Here's how the part is built. I have some questions about the finished solid (model axes, mm). Face numbers are marked on the shaded views. A direction names the side the tool comes from. Give positions to 0.01 mm unless a question says otherwise; leave off trailing zeros. Loops run counter-clockwise (first coordinate to the right, second up) from the corner with the lowest first, then second, coordinate; pieces in that order, holes last. Notation, with made-up numbers: (-5.5, 14.25) - (29.5, 14.25) arc R25 cw to (29.5, 29.25) - close; hole circle Ø3 at (-3, 62.5). An arc over 180 degrees is marked (long way). Put each result on its own line as item: value. Start each with the question number.
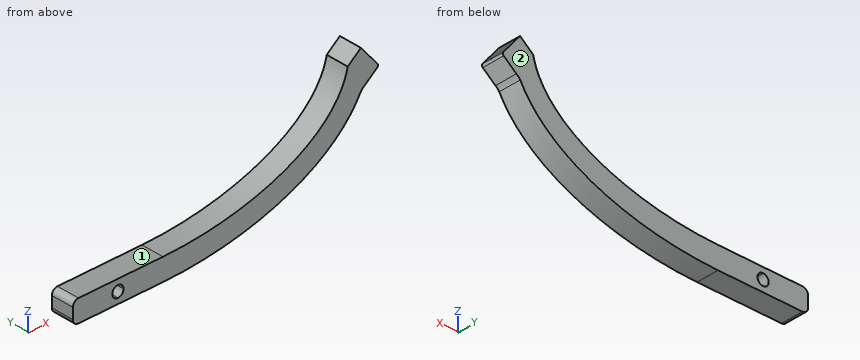
from build123d import *

# Parameters (mm, degrees)
F1_DEPTH = 10


# Not quite as in the source:
# - ends of sketch curves that miss each other by under 0.0002 mm in the source are joined
# - the dataset's text gives a spline's control points without its knots; the knots are read off the source's solid


with BuildPart() as f1:
    # F0 (on Front) → F1 (new body)
    with BuildSketch(Plane.XZ):
        with BuildLine():
            Line((-65.2858525045, 19.1747198819), (-82.7858525045, 19.1747198819))
            ThreePointArc((-82.7858525045, 19.1747198819), (-84.5536194575, 18.4424868349), (-85.2858525045, 16.6747198819))
            Line((-85.2858525045, 16.6747198819), (-85.2858525045, 11.9747207331))
            ThreePointArc((-85.2858525045, 11.9747207331), (-84.5536194575, 10.2069537801), (-82.7858525045, 9.4747207331))
            Line((-82.7858525045, 9.4747207331), (-65.2858525045, 9.4747207331))
            Line((-65.2858525045, 9.4747207331), (-65.2858525045, 11.8247203075))
            ThreePointArc((-65.2858525045, 11.8247203075), (-67.7858525045, 14.3247203075), (-65.2858525045, 16.8247203075))
            Line((-65.2858525045, 16.8247203075), (-65.2858525045, 19.1747198819))
        make_face()
        with BuildLine():
            Line((-45.2858542078, 19.1747198819), (-65.2858525045, 19.1747198819))
            Line((-65.2858525045, 19.1747198819), (-65.2858525045, 16.8247203075))
            ThreePointArc((-65.2858525045, 16.8247203075), (-63.5180855515, 16.0924872605), (-62.7858525045, 14.3247203075))
            ThreePointArc((-62.7858525045, 14.3247203075), (-63.5180855515, 12.5569533545), (-65.2858525045, 11.8247203075))
            Line((-65.2858525045, 11.8247203075), (-65.2858525045, 9.4747207331))
            Line((-65.2858525045, 9.4747207331), (-45.2858525045, 9.4747207331))
            Line((-45.2858525045, 9.4747207331), (-45.2858542078, 19.1747198819))
        make_face()
        with BuildLine():
            add(Edge.make_bspline(
                [(-45.2858542078, 19.1747198819), (-7.4020708747, 19.1747265342), (31.6102094948, 32.6948724687), (36.8064381182, 57.2929121554)],
                knots=[0, 0, 0, 0, 90.5104471403, 90.5104471403, 90.5104471403, 90.5104471403], degree=3))
            Line((-45.2858542078, 19.1747198819), (-45.2858525045, 9.4747207331))
            add(Edge.make_bspline(
                [(-45.2858525045, 9.4747207331), (-40.2618978901, 9.4747216153), (-30.1894784684, 9.9223917761), (-15.362918013, 11.9100905112), (-1.1709415961, 15.2094571968), (12.0418148644, 19.8491680066), (21.9570020274, 24.9039048155), (29.047465051, 29.7583646646), (33.8850587667, 33.8431124408), (38.1663250739, 38.413322434), (40.9420261226, 42.3174471625), (42.2861221075, 44.6734195955), (42.5837097689, 45.2249895308)],
                knots=[0, 0, 0, 0, 0.125, 0.25, 0.375, 0.5, 0.625, 0.6875, 0.75, 0.8125, 0.875, 0.8937572345, 0.8937572345, 0.8937572345, 0.8937572345], degree=3))
            add(Edge.make_bspline(
                [(42.5837097689, 45.2249895308), (42.9712246909, 45.9432369861), (43.3372375793, 46.6745796576), (43.6802036603, 47.4185139687)],
                knots=[0.8937572345, 0.8937572345, 0.8937572345, 0.8937572345, 0.9181826701, 0.9181826701, 0.9181826701, 0.9181826701], degree=3))
            Line((43.6802036603, 47.4185139687), (44.295853648, 46.8606554446))
            Line((44.295853648, 46.8606554446), (49.9209338751, 51.373229087))
            ThreePointArc((49.9209338751, 51.373229087), (50.2893303324, 52.0452304101), (50.0738615656, 52.7806724123))
            Line((50.0738615656, 52.7806724123), (42.6465372943, 61.9985727481))
            Line((42.6465372943, 61.9985727481), (36.8064381182, 57.2929121554))
        make_face()
        with BuildLine():
            add(Edge.make_bspline(
                [(42.5837097689, 45.2249895308), (42.9712246909, 45.9432369861), (43.3372375793, 46.6745796576), (43.6802036603, 47.4185139687)],
                knots=[0.8937572345, 0.8937572345, 0.8937572345, 0.8937572345, 0.9181826701, 0.9181826701, 0.9181826701, 0.9181826701], degree=3))
            add(Edge.make_bspline(
                [(42.5837097689, 45.2249895308), (42.9444412623, 45.4831122336), (42.9444412623, 45.9540075538), (44.295853648, 46.8606554446)],
                knots=[0, 0, 0, 0, 2.3678540998, 2.3678540998, 2.3678540998, 2.3678540998], degree=3))
            Line((44.295853648, 46.8606554446), (43.6802036603, 47.4185139687))
        make_face()
    extrude(amount=F1_DEPTH)


solid = f1.part
1) I'm going to push flat-ended pins straight in: P1, Ø3, axis at x = 23, y = -2.5, coming from the +Z side; P2, Ø5, axis at x = -70.5, y = -5.5, coming from the +Z side; P3, Ø1, axis at y = -3, z = 18.5, coming from the -X side. Where does each tip first touch, or does it pass through?
2) Which directions (+Z, -Z, +X, -X, +Y, -Y) give clear straight access to the entire face, cutting with the end or side of a thin tool? Please do the marked faces 1 and 2.
3) Suppose I cut it at A-A on x = -64. Please give me the cut outline in (y, z).
4) I need wall thicknesses on line 1 (Z direction, x = -73, y = -8); line 2 (Z direction, x = 37, y = -5.5); line 3 (X direction, y = -1.75, z = 36.5). Which ranges of each line are inside material? Lowest first, please.
5) Suppose I cut it at B-B on x = -49.5. Please give me the cut outline in (y, z).
Ans:
1. P1: stops at z = 38.66
1. P2: stops at z = 19.17
1. P3: stops at x = -84.91
2. face 1: +Z, -X, +Y, -Y
2. face 2: +Z, -Z, +X, -X, +Y
3. outline: (-10, 9.47) - (0, 9.47) - (0, 12.18) - (-10, 12.18) - close; (-10, 16.47) - (0, 16.47) - (0, 19.17) - (-10, 19.17) - close
4. line 1: z = 9.47 to 19.17
4. line 2: z = 37.25 to 57.45
4. line 3: x = 21.66 to 36.32
5. outline: (-10, 9.47) - (0, 9.47) - (0, 19.17) - (-10, 19.17) - close
